```python
from build123d import *

# Parameters (mm, degrees)
F1_DEPTH = 3
F4_DEPTH = 10


# Not quite as in the source:
# - a feature names something its author has since deleted; it is built from what else it names


with BuildPart() as f1:
    # F0 (on Top) → F1 (new body)
    with BuildSketch(Plane.XY):
        Polygon((0, -16), (0, 0), (-219, 0), (-219, 3.8), (-222.0407651073, 15.5), (-225.7, 20), (-225.7, 3.8), (-232, 3.8), (-232, -19.5), (-224.5, -49.8), (-218.3, -56), (-218.3, -27), (-218, -27), (-218, -16), align=None)
    extrude(amount=F1_DEPTH)

    # F3 (on offset) → F4 (cut)
    with BuildSketch(Plane.XZ.offset(53)):
        Polygon((-221.3, 3), (-218.3, 1.5), (-221.3, 0), (-213.3, 0), (-213.3, 3), align=None)
    extrude(amount=-F4_DEPTH, mode=Mode.SUBTRACT)


solid = f1.part
```
For this review, take the finished solid that the model builds, in its own axes (mm). Round coordinates to 2 decimals unless told otherwise and drop trailing zeros. Write each loop counter-clockwise with the first axis right and the second up, starting at its lowest first coordinate (ties: lowest second). Pieces come first, ordered by that corner, then holes. Notation, with made-up numbers: M 60.5,81.25 L 71.5,81.25 A35 ccw 71.5,115.25 Z; hole C 25,-22 d7. An arc over 180 degrees is marked long. One line per item, written item: value. Start each with the question number.
(1) We need section A-A (z = 0.7). Give the boundary of the cut face in (x, y).
(2) Wall thickness on line 1 (Y direction, x = -14, z = 1.55); line 2 (X direction, y = 0.5, z = 2); line 3 (X direction, y = -43.5, z = 1.4): over which ranges is each line inside the solid? List them lowest first.
(3) We need section C-C (y = 10). Give the boundary of the cut face in (x, z).
(4) Insertion check: pin 1 (1.5 mm diameter, centred on x = -74.5, z = 2, fed in from -Y); pin 2 (0.9 mm diameter, centred on y = -55, z = 1, fed in from +X); pin 3 (0.9 mm diameter, centred on x = -135, z = 1.5, fed in from +Y). Each pin has a flat end and moves straight along its axis. Give the tip position at first contact, or say it passes through.
(5) We need section D-D (y = -47). Give the boundary of the cut face in (x, z), and give its area (3 significant figures).
(6) We need section B-B (x = -157). Give the boundary of the cut face in (y, z), and give its area (3 significant figures).
Result:
1. outline: M -232,-19.5 L -224.5,-49.8 L -218.3,-56 L -218.3,-53 L -219.9,-53 L -219.9,-43 L -218.3,-43 L -218.3,-27 L -218,-27 L -218,-16 L 0,-16 L 0,0 L -219,0 L -219,3.8 L -222.04,15.5 L -225.7,20 L -225.7,3.8 L -232,3.8 Z
2. line 1: -16 to 0
2. line 2: -232 to -219
2. line 3: -226.06 to -218.5
3. outline: M -225.7,0 L -220.61,0 L -220.61,3 L -225.7,3 Z
4. pin 1: y = -16
4. pin 2: x = -218.3
4. pin 3: y = 0
5. outline: M -225.19,0 L -221.3,0 L -218.3,1.5 L -221.3,3 L -225.19,3 Z
5. area: 16.2 mm²
6. outline: M -16,0 L 0,0 L 0,3 L -16,3 Z
6. area: 48.0 mm²
